from build123d import *

# Parameters (mm, degrees)
F1_DEPTH = 1
F2_W     = 46.682928
F2_H     = 30
F3_DEPTH = 1
F5_DEPTH = 2
F7_DEPTH = 2


with BuildPart() as f1:
    # F0 (on Front) → F1 (new body)
    with BuildSketch(Plane.XZ):
        with BuildLine():
            Line((-63.739401, 25.876286), (-63.739401, 24.876286))
            Line((-63.739401, 24.876286), (-53.739401, 24.876286))
            ThreePointArc((-53.739401, 24.876286), (-45.845818, 21.914612), (-41.848604, 14.49151))
            Line((-41.848604, 14.49151), (-41.848604, -5.344726))
            ThreePointArc((-41.848604, -5.344726), (-48.443242, -13.888168), (-58.739401, -17.123714))
            Line((-58.739401, -17.123714), (-63.739401, -17.123714))
            Line((-63.739401, -17.123714), (-63.739401, -18.123714))
            Line((-63.739401, -18.123714), (-58.739401, -18.123714))
            ThreePointArc((-58.739401, -18.123714), (-47.797274, -14.656578), (-40.848604, -5.520541))
            Line((-40.848604, -5.520541), (-40.848604, 14.55776))
            ThreePointArc((-40.848604, 14.55776), (-45.162081, 22.645092), (-53.739401, 25.876286))
            Line((-53.739401, 25.876286), (-63.739401, 25.876286))
        make_face()
    extrude(amount=F1_DEPTH)

    # F2 (on face) → F3 (join)
    with BuildSketch(Plane.YZ.offset(-40.848604)):
        with Locations((5.529391, 3)):
            Rectangle(F2_W, F2_H)
    extrude(amount=F3_DEPTH)

    # F4 (on face) → F5 (join)
    with BuildSketch(Plane(origin=(0, 28.870855, 0), x_dir=(-1, 0, 0), z_dir=(0, 1, 0))):
        with BuildLine():
            Line((62.989129, 21.67293), (62.989129, 22.67293))
            Line((62.989129, 22.67293), (52.540804, 22.67293))
            ThreePointArc((52.540804, 22.67293), (44.763407, 20.089843), (40.076731, 13.367097))
            Line((40.076731, 13.367097), (40.076731, -6.663155))
            ThreePointArc((40.076731, -6.663155), (47.020666, -15.841348), (57.989129, -19.32707))
            Line((57.989129, -19.32707), (62.989129, -19.32707))
            Line((62.989129, -19.32707), (62.989129, -18.32707))
            Line((62.989129, -18.32707), (57.989129, -18.32707))
            ThreePointArc((57.989129, -18.32707), (47.667229, -15.073541), (41.076731, -6.489113))
            Line((41.076731, -6.489113), (41.076731, 13.219057))
            ThreePointArc((41.076731, 13.219057), (45.418779, 19.330919), (52.540804, 21.67293))
            Line((52.540804, 21.67293), (62.989129, 21.67293))
        make_face()
    extrude(amount=-F5_DEPTH)

    # F6 (on face) → F7 (join)
    with BuildSketch(Plane.XZ.offset(17.812073)):
        with BuildLine():
            Line((-62.944316, 24.917709), (-62.944316, 23.917709))
            Line((-62.944316, 23.917709), (-52.944316, 23.917709))
            ThreePointArc((-52.944316, 23.917709), (-45.050733, 20.956036), (-41.053519, 13.532934))
            Line((-41.053519, 13.532934), (-41.053519, -6.303302))
            ThreePointArc((-41.053519, -6.303302), (-47.648157, -14.846744), (-57.944316, -18.082291))
            Line((-57.944316, -18.082291), (-62.944316, -18.082291))
            Line((-62.944316, -18.082291), (-62.944316, -19.082291))
            Line((-62.944316, -19.082291), (-57.944316, -19.082291))
            ThreePointArc((-57.944316, -19.082291), (-47.002189, -15.615154), (-40.053519, -6.479117))
            Line((-40.053519, -6.479117), (-40.053519, 13.599184))
            ThreePointArc((-40.053519, 13.599184), (-44.366996, 21.686516), (-52.944316, 24.917709))
            Line((-52.944316, 24.917709), (-62.944316, 24.917709))
        make_face()
    extrude(amount=-F7_DEPTH)


solid = f1.part
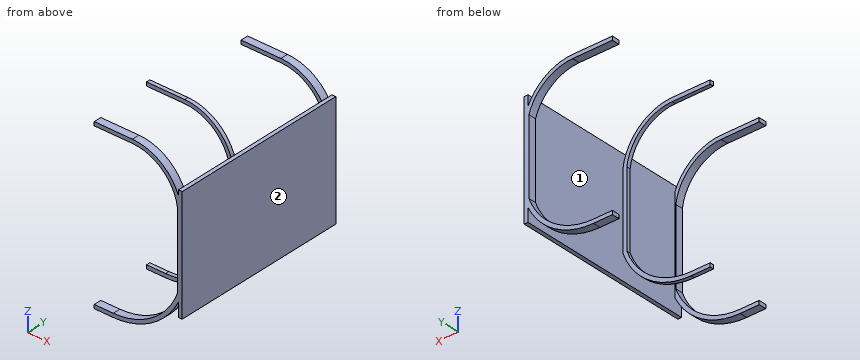
The listing builds one solid part. Answer for the finished solid, in the listing's coordinates (mm). Face numbers are marked on the shaded views. Give positions to 0.01 mm unless a question says otherwise; leave off trailing zeros. Loops run counter-clockwise (first coordinate to the right, second up) from the corner with the lowest first, then second, coordinate; pieces in that order, holes last. Notation, with made-up numbers: (1, -33) - (27, -33) arc R10 ccw to (27, -21) - close; hole circle Ø8 at (34.25, 26.25). An arc over 180 degrees is marked (long way). Use one line per item in the form item = value.
1. The mould has two halves that part along Y. Classify the marked faces 1 and 2: pulls with the +Y half, pulls with the -Y half, needs draft (parallel to the pull), parting line crosses it, or undercut.
Calculated:
face_1 = undercut
face_2 = needs draft
2. Section D-D on z = 20 is taken. Give the vertices of the cut face in (x, y) (1 decimal).
Calculated:
outline = (-46.4, 26.9) - (-44.6, 26.9) - (-44.6, 28.9) - (-46.4, 28.9) - close; (-44.1, -17.8) - (-42.8, -17.8) - (-42.8, -15.8) - (-44.1, -15.8) - close; (-44.1, -1) - (-42.9, -1) - (-42.9, 0) - (-44.1, 0) - close
3. Section A-A on z = 0 is taken. Give the vertices of the cut face in (x, y).
Calculated:
outline = (-41.85, -1) - (-40.85, -1) - (-40.85, -15.81) - (-41.05, -15.81) - (-41.05, -17.81) - (-39.85, -17.81) - (-39.85, 28.87) - (-41.08, 28.87) - (-41.08, 26.87) - (-40.85, 26.87) - (-40.85, 0) - (-41.85, 0) - close
4. Given pin 1 Ø0.8 at (y, z) = (-16.5, -18.5) entering from -X; pin 2 Ø11.5 at (x, z) = (-52, 6) entering from +Y; pin 3 Ø1 at (y, z) = (-16.5, 4.5) entering from -X; pin 4 Ø0.5 at (y, z) = (-0.5, 3) entering from -X, each flat-ended and moving along its own axis, determine where each tip first touches the part or whether it passes through.
Calculated:
pin_1 = -62.94
pin_2 = through
pin_3 = -41.05
pin_4 = -41.85
5. Section C-C on z = -11 is taken. Give the vertices of the cut face in (x, y), then the cut area to 3 significant figures.
Calculated:
outline = (-45.21, -1) - (-43.91, -1) - (-43.91, 0) - (-45.21, 0) - close; (-43.63, -17.81) - (-42.39, -17.81) - (-42.39, -15.81) - (-43.63, -15.81) - close; (-43.49, 26.87) - (-42.27, 26.87) - (-42.27, 28.87) - (-43.49, 28.87) - close; (-40.85, -17.81) - (-39.85, -17.81) - (-39.85, 28.87) - (-40.85, 28.87) - close
area = 52.9 mm^2
6. Find the intervals of material crossed by line 1 along X through (y, z) = (25, -2); line 2 along Z through (x, y) = (-52.25, -0.5); line 3 along X through (y, z) = (27.5, -13.5), in increasing order. Write a range as [from, to].
Calculated:
line_1 = [-40.85, -39.85]
line_2 = [-16.98, -15.91], [24.78, 25.79]
line_3 = [-45.72, -44.3]
7. Section B-B on x = -50.75 is taken. Give the vertices of the cut face in (y, z), then the cut area to 3 significant figures.
Calculated:
outline = (-17.81, -17.67) - (-15.81, -17.67) - (-15.81, -16.58) - (-17.81, -16.58) - close; (-17.81, 23.72) - (-15.81, 23.72) - (-15.81, 24.73) - (-17.81, 24.73) - close; (-1, -16.36) - (0, -16.36) - (0, -15.25) - (-1, -15.25) - close; (-1, 24.5) - (0, 24.5) - (0, 25.53) - (-1, 25.53) - close; (26.87, -17.89) - (28.87, -17.89) - (28.87, -16.81) - (26.87, -16.81) - close; (26.87, 21.54) - (28.87, 21.54) - (28.87, 22.55) - (26.87, 22.55) - close
area = 10.5 mm^2
